Geometry: see drawing. Coordinates: mm, zero at the bounding-box minimum. A direction names the side the tool comes from. Give positions to 0.01 mm unless a question says otherwise; leave off trailing zeros. Write each loop counter-clockwise with the first axis right and the second up, starting at its lowest first coordinate (ties: lowest second). Pieces come first, ordered by that corner, then holes. Notation, with made-up numbers: M -13.5,37.5 L 42.5,37.5 A24 cw 42.5,63.5 Z; hole C 5,-16.5 d1. An arc over 180 degrees is marked long. Use a Markdown table: item, result. Add a question column.
(1) Cut plane D-D (y = 4.5). Output: boundary loops of the cut face in (x, z), plus the area to 3 significant figures.
(2) Cut plane C-C (z = 25). Output: boundary loops of the cut face in (x, y).
(3) Cut plane A-A (y = 2). Output: boundary loops of the cut face in (x, z).
(4) Cut plane B-B (x = 2.6). Output: boundary loops of the cut face in (y, z).
(5) Reachability of the marked faces 1, 2 and 3 from +Z, -Z, +X, -X, +Y, -Y: full face, straight path, thin tool, end or side. Return the list, or none.
(6) Pin query (flat end, axial travel): pin 1 Ø1 at (x, y) = (2, 3.5) entering from +Z; pin 2 Ø1.5 at (x, z) = (1, 3.5) entering from +Y; pin 3 Ø2.5 at (y, z) = (8.11, 31.22) entering from -X. Return the tip coordinate at first contact, or that it passes through.
(7) Material intervals for L1, parallel to Y at x = 0.7, z = 2; L2, parallel to Y at x = 0.85, z = 27; L3, parallel to Y at x = 1.3, z = 14, sorted ascending.
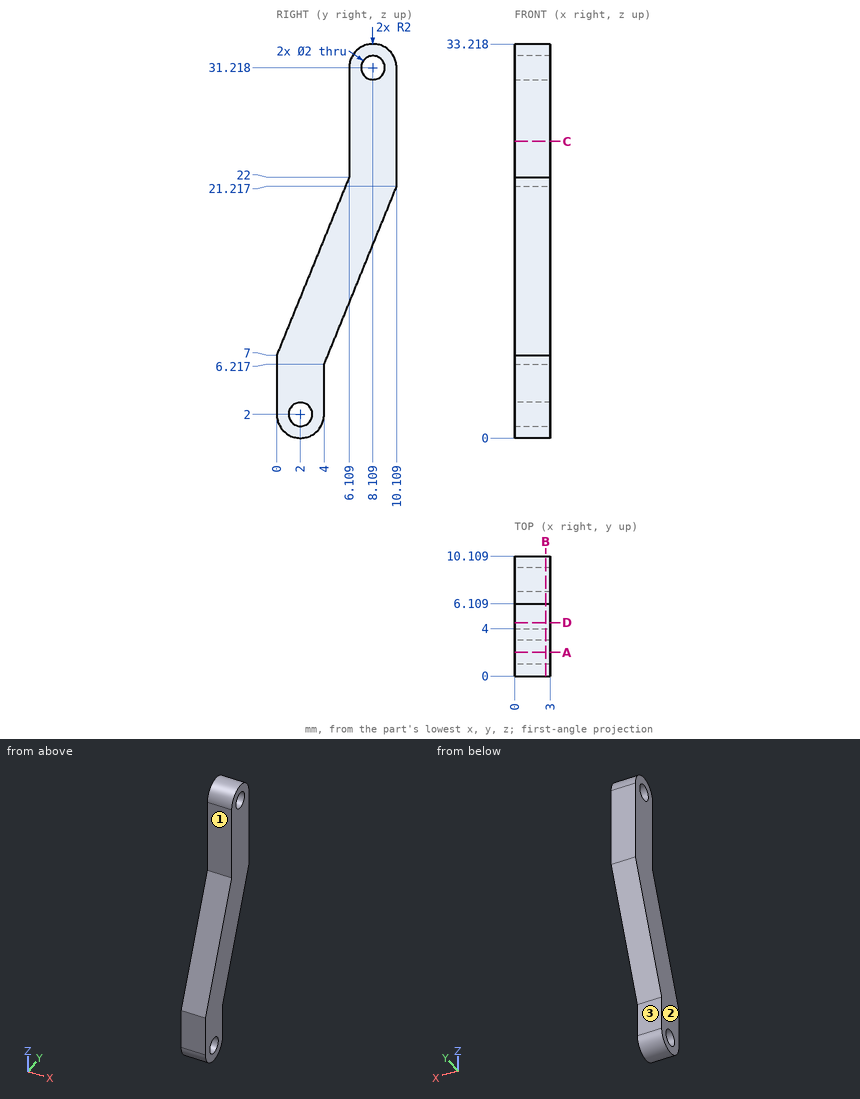
Answer list:
| question | item | result |
|---|---|---|
| 1 | outline | M 0,7.44 L 3,7.44 L 3,18.05 L 0,18.05 Z |
| 1 | area | 31.8 mm² |
| 2 | outline | M 0,6.11 L 3,6.11 L 3,10.11 L 0,10.11 Z |
| 3 | outline | M 0,0 L 3,0 L 3,1 L 0,1 Z; M 0,3 L 3,3 L 3,11.91 L 0,11.91 Z |
| 4 | outline | M 0,2 A2 ccw 4,2 L 4,6.22 L 10.11,21.22 L 10.11,31.22 A2 ccw 6.11,31.22 L 6.11,22 L 0,7 Z; hole C 2,2 d2; hole C 8.11,31.22 d2 |
| 5 | face 1 | +Z, +X, -X, -Y |
| 5 | face 2 | +Z, -Z, -X, +Y, -Y |
| 5 | face 3 | -Z, +X, -X, +Y |
| 6 | pin 1 | z = 16.82 |
| 6 | pin 2 | y = 4 |
| 6 | pin 3 | x = 0 |
| 7 | L1 | 0 to 1, 3 to 4 |
| 7 | L2 | 6.11 to 10.11 |
| 7 | L3 | 2.85 to 7.17 |
